from build123d import *

# Parameters (mm, degrees)
F0_R      = 20
F1_DEPTH  = 1672
F2_R      = 75
F3_DEPTH  = 6
F5_R      = 23.5
F6_DEPTH  = 48
F7_R      = 0.5
F8_R      = 1
F9_W      = 12
F9_H      = 5
F10_DEPTH = 45
F11_R     = 4.99999
F12_SIZE2 = 1
F12_SIZE  = 1


# Not quite as in the source:
# - a fillet or chamfer is up to 0.001 mm smaller than in the source, because OpenCascade refuses the exact size


with BuildPart() as f1:
    # F0 (on Top) → F1 (new body)
    with BuildSketch(Plane.XY):
        Circle(F0_R)
    extrude(amount=F1_DEPTH)

    # F2 (on face) → F3 (join)
    with BuildSketch(Plane(origin=(0, 0, 0), x_dir=(1, 0, 0), z_dir=(0, 0, -1))):
        Circle(F2_R)
    extrude(amount=F3_DEPTH)

    # F5 (on offset) → F6 (join)
    with BuildSketch(Plane.XY.offset(1569.91401)):
        Circle(F5_R)
    extrude(amount=F6_DEPTH)

    # F7
    f7_edges = [f1.edges().sort_by_distance(p)[0] for p in [
        (-20, 0, 1617.91401),
    ]]
    fillet(f7_edges, radius=F7_R)

    # F8
    f8_edges = [f1.edges().sort_by_distance(p)[0] for p in [
        (-20, 0, 1569.91401),
    ]]
    fillet(f8_edges, radius=F8_R)

    # F9 (on face) → F10 (cut)
    with BuildSketch(Plane.XY.offset(1672)):
        with Locations((0, 17.5)):
            Rectangle(F9_W, F9_H)
    extrude(amount=-F10_DEPTH, mode=Mode.SUBTRACT)

    # F11 (radius 5 in the source; OpenCascade refuses exactly that, so slightly less here)
    f11_edges = [f1.edges().sort_by_distance(p)[0] for p in [
        (0, 15, 1627),
    ]]
    fillet(f11_edges, radius=F11_R)

    # F12
    f12_edges = [f1.edges().sort_by_distance(p)[0] for p in [
        (-11.83216, -16.124515, 1672),
    ]]
    chamfer(f12_edges, length=F12_SIZE, length2=F12_SIZE2)


solid = f1.part
Read the model definition and answer for the solid it produces. Units are mm, in the model's axes. A direction names the side the tool comes from. Coordinates: 2 decimals unless noted, no trailing zeros. Loops run counter-clockwise (first coordinate to the right, second up) from the corner with the lowest first, then second, coordinate; pieces in that order, holes last. Notation, with made-up numbers: (25, 27.5) -> (45, 27.5) arc R17 cw to (45, 44.5) -> close; hole circle Ø6 at (10.25, 68). An arc over 180 degrees is marked (long way). Answer in a Markdown table with one row per item.
Item 1: Each of these flat-tipped pins is pushed along its axis until it touches: P1, Ø6, axis at x = -2.5, z = 1648.5, coming from the +Y side; P2, Ø1.5, axis at x = -17.5, y = 59.5, coming from the +Z side; P3, Ø4, axis at x = -2.5, z = 1181.5, coming from the +Y side. Where does it stop, or does it pass through?
Returned:
| item | result |
|---|---|
| P1 | stops at y = 15 |
| P2 | stops at z = 0 |
| P3 | stops at y = 19.99 |
Item 2: A cutting plane is placed at A-A on y = 0. Determine the outline of the cut face in (x, z).
Returned:
| item | result |
|---|---|
| outline | (-75, -6) -> (75, -6) -> (75, 0) -> (20, 0) -> (20, 1568.91) arc R1 cw to (21, 1569.91) -> (23.5, 1569.91) -> (23.5, 1617.91) -> (20.5, 1617.91) arc R0.5 cw to (20, 1618.41) -> (20, 1671) -> (19, 1672) -> (-19, 1672) -> (-20, 1671) -> (-20, 1618.41) arc R0.5 cw to (-20.5, 1617.91) -> (-23.5, 1617.91) -> (-23.5, 1569.91) -> (-21, 1569.91) arc R1 cw to (-20, 1568.91) -> (-20, 0) -> (-75, 0) -> close |
Item 3: Straight lines are drawn through the part: line 1 along Z through (x, y) = (9, 19); line 2 along Z through (x, y) = (-53, -23); line 3 along Z through (x, y) = (-15, -12). For each, find the intervals that lie inside material, in ascending order. Write a range as [from, to].
Returned:
| item | result |
|---|---|
| line 1 | z = [-6, 0], [1569.91, 1617.91] |
| line 2 | z = [-6, 0] |
| line 3 | z = [-6, 1671.79] |
Item 4: A cutting plane is placed at B-B on z = 959.5. Determine the outline of the cut face in (x, y).
Returned:
| item | result |
|---|---|
| outline | circle Ø40 at (0, 0) |
Item 5: For faces 1 (the flat face through (-1, -1, -6)), 2 (the flat face through (2, 21, 1617.914)), 3 (the cylindrical face through (-4.336, -19.524, 773.475)), determine the directions among +Z, -Z, +X, -X, +Y, -Y from which every point of the face is accessible in a straight line to the end or side of a thin tool.
Returned:
| item | result |
|---|---|
| face 1 | -Z, +X, -X, +Y, -Y |
| face 2 | +Z |
| face 3 | none |
Item 6: A cutting plane is placed at C-C on x = 57. Determine the outline of the cut face in (y, z).
Returned:
| item | result |
|---|---|
| outline | (-48.74, -6) -> (48.74, -6) -> (48.74, 0) -> (-48.74, 0) -> close |
Item 7: For a pull along Z with two mould halves and no side action, classify faces 4 (the conical face through (-0.761, -19.145, 1671.84)), 5 (the cylindrical face through (-9.764, -74.362, -2.958)), 6 (the flat face through (-18, -12, 1569.914)) as released by +Z, released by -Z, zero draft, split by the parting line, or undercut.
Returned:
| item | result |
|---|---|
| face 4 | released by +Z |
| face 5 | zero draft |
| face 6 | undercut |
